CAD build for the part. Positions are in the model's coordinates, mm. Face numbers are marked on the shaded views. A direction names the side the tool comes from. Coordinates: 2 decimals unless noted, no trailing zeros. Loops run counter-clockwise (first coordinate to the right, second up) from the corner with the lowest first, then second, coordinate; pieces in that order, holes last. Notation, with made-up numbers: M 66.5,-19 L 108.5,-19 A24 ccw 108.5,18 Z; hole C -2.5,-2.5 d7. An arc over 180 degrees is marked long. Answer as a JSON object with one key per item and string values. Group by question number.
```python
from build123d import *

# Parameters (mm, degrees)
SKETCH1_W               = 27
SKETCH1_H               = 13.8
SKETCH1_W_2             = 21
SKETCH1_H_2             = 7.8
BOSS_EXTRUDE1_DEPTH     = 22
SKETCH3_W               = 21
SKETCH3_H               = 7.8
BOSS_EXTRUDE2_DEPTH     = 2
SKETCH6_W               = 27
SKETCH6_H               = 13.8
BOSS_EXTRUDE3_DEPTH     = 2
SKETCH8_R               = 3
CUT_EXTRUDE2_DEPTH      = 5
CUT_EXTRUDE3_DEPTH      = 45
CUT_EXTRUDE5_DEPTH      = 45
CUT_EXTRUDE5_DEPTH_BACK = 45
SKETCH7_R               = 1.5
CUT_EXTRUDE6_DEPTH      = 4.10483504
CUT_EXTRUDE6_DEPTH_BACK = 17.904835039
SKETCH15_W              = 4.518403315
SKETCH15_H              = 4.307078744
CUT_EXTRUDE7_DEPTH      = 10
CUT_EXTRUDE7_DEPTH_BACK = 20


with BuildPart() as part:
    # Sketch1 → Boss-Extrude1 (new body)
    with BuildSketch(Plane(origin=(0, 0, 0), x_dir=(1, 0, 0), z_dir=(0, 1, 0))):
        with Locations((10.5, 3.9)):
            Rectangle(SKETCH1_W, SKETCH1_H)
        with Locations((10.5, 3.9)):
            Rectangle(SKETCH1_W_2, SKETCH1_H_2, mode=Mode.SUBTRACT)
    extrude(amount=BOSS_EXTRUDE1_DEPTH)

    # Sketch3 → Boss-Extrude2 (add)
    with BuildSketch(Plane(origin=(0, 22, 0), x_dir=(1, 0, 0), z_dir=(0, 1, 0))):
        with Locations((10.5, 3.9)):
            Rectangle(SKETCH3_W, SKETCH3_H)
    extrude(amount=-BOSS_EXTRUDE2_DEPTH)

    # Sketch6 → Boss-Extrude3 (add)
    with BuildSketch(Plane.XZ):
        with BuildLine():
            Line((-6, 2.2), (-6, -10))
            ThreePointArc((-6, -10), (-5.19544984, -12.99544984), (-2.2, -13.8))
            Line((-2.2, -13.8), (23.2, -13.8))
            ThreePointArc((23.2, -13.8), (26.19544984, -12.99544984), (27, -10))
            Line((27, -10), (27, 2.2))
            ThreePointArc((27, 2.2), (26.19544984, 5.19544984), (23.2, 6))
            Line((23.2, 6), (-2.2, 6))
            ThreePointArc((-2.2, 6), (-5.19544984, 5.19544984), (-6, 2.2))
        make_face()
        with Locations((10.5, -3.9)):
            Rectangle(SKETCH6_W, SKETCH6_H, mode=Mode.SUBTRACT)
    extrude(amount=-BOSS_EXTRUDE3_DEPTH)

    # Sketch8 → Cut-Extrude2 (cut)
    with BuildSketch(Plane.ZY.offset(3)):
        with Locations((-3.9, 16.816542633)):
            Circle(SKETCH8_R)
    extrude(amount=-CUT_EXTRUDE2_DEPTH, mode=Mode.SUBTRACT)

    # Sketch12 → Cut-Extrude3 (cut)
    with BuildSketch(Plane.ZY.offset(6)):
        with BuildLine():
            Line((3, 2), (6.104834939, 2))
            Line((6.104834939, 2), (6.104834939, 1.56677659))
            add(Edge.make_bspline(
                [(6.104834939, 1.56677659), (4.570942596, 1.898546139), (3, 2)],
                knots=[0, 0, 0, 1, 1, 1], degree=2))
        make_face()
        with BuildLine():
            Line((-13.933772202, 2), (-13.933772202, 1.56677659))
            add(Edge.make_bspline(
                [(-13.933772202, 1.56677659), (-12.399879859, 1.898546139), (-10.828937263, 2)],
                knots=[0, 0, 0, 1, 1, 1], degree=2))
            Line((-10.828937263, 2), (-13.933772202, 2))
        make_face()
    extrude(amount=-CUT_EXTRUDE3_DEPTH, mode=Mode.SUBTRACT)

    # Sketch13 → Cut-Extrude5 (cut, two sides)
    with BuildSketch(Plane(origin=(27, 0, -10), x_dir=(1, 0, 0), z_dir=(0, 0, 1))) as cut_extrude5_sk:
        with BuildLine():
            Line((-3.377880941, 0), (0.509598996, 0))
            Line((0.509598996, 0), (0.509598996, 1.57572602))
            Line((0.509598996, 1.57572602), (0.175576118, 1.57572602))
            add(Edge.make_bspline(
                [(-3.377880941, 0), (-2.337490472, 0.807111843), (-1.090367189, 1.274012221), (0.175576118, 1.57572602)],
                knots=[0, 0, 0, 0, 1, 1, 1, 1], degree=3))
        make_face()
    extrude(amount=CUT_EXTRUDE5_DEPTH, mode=Mode.SUBTRACT)
    extrude(cut_extrude5_sk.sketch, amount=-CUT_EXTRUDE5_DEPTH_BACK, mode=Mode.SUBTRACT)

    # Sketch7 → Cut-Extrude6 (cut, two sides)
    with BuildSketch(Plane(origin=(0, 0, -10.8), x_dir=(-1, 0, 0), z_dir=(0, 0, -1))) as cut_extrude6_sk:
        with Locations((-6.4, 7)):
            Circle(SKETCH7_R)
        with Locations((-15.5, 7)):
            Circle(SKETCH7_R)
    extrude(amount=CUT_EXTRUDE6_DEPTH, mode=Mode.SUBTRACT)
    extrude(cut_extrude6_sk.sketch, amount=-CUT_EXTRUDE6_DEPTH_BACK, mode=Mode.SUBTRACT)

    # Sketch15 → Cut-Extrude7 (cut, two sides)
    with BuildSketch(Plane.XY.offset(3)) as cut_extrude7_sk:
        with Locations((-5.259201658, -0.153539372)):
            Rectangle(SKETCH15_W, SKETCH15_H)
    extrude(amount=CUT_EXTRUDE7_DEPTH, mode=Mode.SUBTRACT)
    extrude(cut_extrude7_sk.sketch, amount=-CUT_EXTRUDE7_DEPTH_BACK, mode=Mode.SUBTRACT)


solid = part.part
```
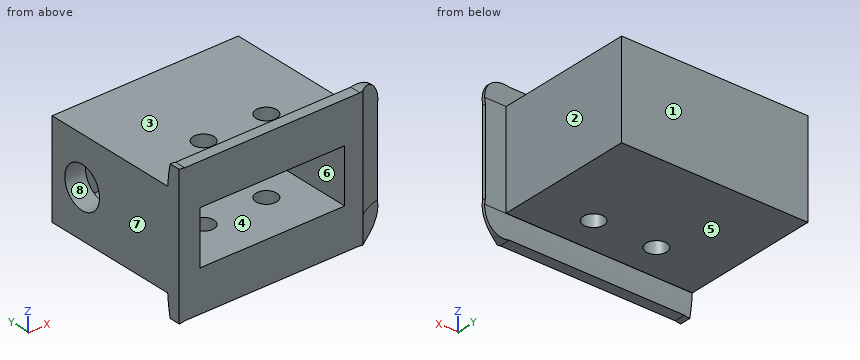
Item 1: Tool access for the marked faces 1, 2, 3 and 4: list every direction of +Z, -Z, +X, -X, +Y, -Y with a clear straight run to the whole face (end or side of a thin tool).
Item 2: Slice it at B-B, the plane x = 6.4. Count the separate pieces of the cut face and the enclosed holes in it, then the cut area to 3 significant figures.
Item 3: Drill centre lines: L1, parallel to Z at x = 17.5, y = 17; L2, parallel to X at y = 12.5, z = -7; L3, parallel to Y at x = -1.85, z = -3.9. Where is each one in solid material? Low to high. Write a range as from..to.
Item 4: Slice it at A-A, the plane y = 7. Write the cut outline in (x, z).
Item 5: Pull direction Z, two halves, no side cores. Call the marked faces 5, 6, 7 and 8: released by +Z, released by -Z, zero draft, split by the parting line, or undercut.
Item 6: Pin check, flat tips, straight feed: pin 1 (8 mm diameter, centred on x = 10, y = 9, fed in from +Z); pin 2 (10 mm diameter, centred on x = 8.5, y = 2.5, fed in from -Z); pin 3 (0.5 mm diameter, centred on x = 12.5, y = 1, fed in from +Z); pin 4 (2.5 mm diameter, centred on x = 15.5, y = 7, fed in from +Z). Stop position of each tip, or through.
Computed:
{
 "1": {"face 1": "+Z, -Z, +X, -X, +Y", "face 2": "+Z, -Z, +X, +Y", "face 3": "+Z, +X, -X, +Y", "face 4": "-Y"},
 "2": {"separate pieces": "3", "enclosed holes": "0", "area": "141 mm2"},
 "3": {"L1": "-10.8..-7.8, 0..3", "L2": "-3..0, 21..24", "L3": "0..13.82, 19.82..22"},
 "4": {"outline": "M -3,-10.8 L 4.9,-10.8 L 4.9,-7.8 L 0,-7.8 L 0,0 L 4.9,0 L 4.9,3 L -3,3 Z; M 7.9,-10.8 L 14,-10.8 L 14,-7.8 L 7.9,-7.8 Z; M 7.9,0 L 14,0 L 14,3 L 7.9,3 Z; M 17,-10.8 L 24,-10.8 L 24,3 L 17,3 L 17,0 L 21,0 L 21,-7.8 L 17,-7.8 Z"},
 "5": {"face 5": "released by -Z", "face 6": "undercut", "face 7": "zero draft", "face 8": "undercut"},
 "6": {"pin 1": "z = 3", "pin 2": "z = -13.8", "pin 3": "z = 6", "pin 4": "through"}
}
